from build123d import *

# Parameters (mm, degrees)
F0_R     = 4.7575
F0_R_2   = 1.5
F1_DEPTH = 3


with BuildPart() as f1:
    # F0 (on Front) → F1 (new body)
    with BuildSketch(Plane.XZ):
        with BuildLine():
            ThreePointArc((20.795049, 31.12199), (16.264046, 39.26488), (7.30225, 36.71089))
            ThreePointArc((7.30225, 36.71089), (4.659309, 40.877145), (0, 42.5))
            ThreePointArc((0, 42.5), (-4.659309, 40.877145), (-7.30225, 36.71089))
            ThreePointArc((-7.30225, 36.71089), (-16.264046, 39.26488), (-20.795049, 31.12199))
            ThreePointArc((-20.795049, 31.12199), (-25.609878, 32.199136), (-30.052038, 30.052038))
            ThreePointArc((-30.052038, 30.052038), (-32.199136, 25.609878), (-31.12199, 20.795049))
            ThreePointArc((-31.12199, 20.795049), (-39.26488, 16.264046), (-36.71089, 7.30225))
            ThreePointArc((-36.71089, 7.30225), (-40.877145, 4.659309), (-42.5, 0))
            ThreePointArc((-42.5, 0), (-40.877145, -4.659309), (-36.71089, -7.30225))
            ThreePointArc((-36.71089, -7.30225), (-39.26488, -16.264046), (-31.12199, -20.795049))
            ThreePointArc((-31.12199, -20.795049), (-32.199136, -25.609878), (-30.052038, -30.052038))
            ThreePointArc((-30.052038, -30.052038), (-25.609878, -32.199136), (-20.795049, -31.12199))
            ThreePointArc((-20.795049, -31.12199), (-16.264046, -39.26488), (-7.30225, -36.71089))
            ThreePointArc((-7.30225, -36.71089), (-4.659309, -40.877145), (0, -42.5))
            ThreePointArc((0, -42.5), (4.659309, -40.877145), (7.30225, -36.71089))
            ThreePointArc((7.30225, -36.71089), (16.264046, -39.26488), (20.795049, -31.12199))
            ThreePointArc((20.795049, -31.12199), (25.609878, -32.199136), (30.052038, -30.052038))
            ThreePointArc((30.052038, -30.052038), (32.199136, -25.609878), (31.12199, -20.795049))
            ThreePointArc((31.12199, -20.795049), (39.26488, -16.264046), (36.71089, -7.30225))
            ThreePointArc((36.71089, -7.30225), (40.877145, -4.659309), (42.5, 0))
            ThreePointArc((42.5, 0), (40.877145, 4.659309), (36.71089, 7.30225))
            ThreePointArc((36.71089, 7.30225), (39.26488, 16.264046), (31.12199, 20.795049))
            ThreePointArc((31.12199, 20.795049), (32.199136, 25.609878), (30.052038, 30.052038))
            ThreePointArc((30.052038, 30.052038), (25.609878, 32.199136), (20.795049, 31.12199))
        make_face()
        with BuildLine():
            ThreePointArc((-28.112798, -28.112798), (-28.112798, -21.384677), (-21.384677, -21.384677))
            ThreePointArc((-21.384677, -21.384677), (-20.35338, -22.928121), (-19.991237, -24.748737))
            ThreePointArc((-19.991237, -24.748737), (-22.928121, -29.144094), (-28.112798, -28.112798))
        make_face(mode=Mode.SUBTRACT)
        with Locations((-13.39392, -32.335784)):
            Circle(F0_R, mode=Mode.SUBTRACT)
        with Locations((-32.335784, -13.39392)):
            Circle(F0_R, mode=Mode.SUBTRACT)
        with BuildLine():
            ThreePointArc((0, -39.7575), (-4.7575, -35), (0, -30.2425))
            ThreePointArc((0, -30.2425), (3.364061, -31.635939), (4.7575, -35))
            ThreePointArc((4.7575, -35), (3.364061, -38.364061), (0, -39.7575))
        make_face(mode=Mode.SUBTRACT)
        with Locations((13.39392, -32.335784)):
            Circle(F0_R, mode=Mode.SUBTRACT)
        with Locations((0, -27)):
            Circle(F0_R_2, mode=Mode.SUBTRACT)
        with BuildLine():
            ThreePointArc((28.112798, -28.112798), (21.384677, -28.112798), (21.384677, -21.384677))
            ThreePointArc((21.384677, -21.384677), (26.569354, -20.35338), (29.506237, -24.748737))
            ThreePointArc((29.506237, -24.748737), (29.144094, -26.569354), (28.112798, -28.112798))
        make_face(mode=Mode.SUBTRACT)
        with Locations((32.335784, -13.39392)):
            Circle(F0_R, mode=Mode.SUBTRACT)
        with BuildLine():
            ThreePointArc((-39.7575, 0), (-35, 4.7575), (-30.2425, 0))
            ThreePointArc((-30.2425, 0), (-35, -4.7575), (-39.7575, 0))
        make_face(mode=Mode.SUBTRACT)
        with Locations((-27, 0)):
            Circle(F0_R_2, mode=Mode.SUBTRACT)
        with Locations((-32.335784, 13.39392)):
            Circle(F0_R, mode=Mode.SUBTRACT)
        with BuildLine():
            ThreePointArc((-19.991237, 24.748737), (-20.35338, 22.928121), (-21.384677, 21.384677))
            ThreePointArc((-21.384677, 21.384677), (-28.112798, 21.384677), (-28.112798, 28.112798))
            ThreePointArc((-28.112798, 28.112798), (-22.928121, 29.144094), (-19.991237, 24.748737))
        make_face(mode=Mode.SUBTRACT)
        with Locations((-13.39392, 32.335784)):
            Circle(F0_R, mode=Mode.SUBTRACT)
        with BuildLine():
            ThreePointArc((0, 11), (4.209518, 10.162675), (7.778175, 7.778175))
            ThreePointArc((7.778175, 7.778175), (10.162675, 4.209518), (11, 0))
            ThreePointArc((11, 0), (10.162675, -4.209518), (7.778175, -7.778175))
            ThreePointArc((7.778175, -7.778175), (4.209518, -10.162675), (0, -11))
            ThreePointArc((0, -11), (-4.209518, -10.162675), (-7.778175, -7.778175))
            ThreePointArc((-7.778175, -7.778175), (-10.162675, -4.209518), (-11, 0))
            ThreePointArc((-11, 0), (-10.162675, 4.209518), (-7.778175, 7.778175))
            ThreePointArc((-7.778175, 7.778175), (-4.209518, 10.162675), (0, 11))
        make_face(mode=Mode.SUBTRACT)
        with Locations((27, 0)):
            Circle(F0_R_2, mode=Mode.SUBTRACT)
        with BuildLine():
            ThreePointArc((39.7575, 0), (35, -4.7575), (30.2425, 0))
            ThreePointArc((30.2425, 0), (35, 4.7575), (39.7575, 0))
        make_face(mode=Mode.SUBTRACT)
        with Locations((32.335784, 13.39392)):
            Circle(F0_R, mode=Mode.SUBTRACT)
        with Locations((0, 27)):
            Circle(F0_R_2, mode=Mode.SUBTRACT)
        with BuildLine():
            ThreePointArc((0, 39.7575), (3.364061, 38.364061), (4.7575, 35))
            ThreePointArc((4.7575, 35), (3.364061, 31.635939), (0, 30.2425))
            ThreePointArc((0, 30.2425), (-4.7575, 35), (0, 39.7575))
        make_face(mode=Mode.SUBTRACT)
        with Locations((13.39392, 32.335784)):
            Circle(F0_R, mode=Mode.SUBTRACT)
        with BuildLine():
            ThreePointArc((21.384677, 21.384677), (21.384677, 28.112798), (28.112798, 28.112798))
            ThreePointArc((28.112798, 28.112798), (29.144094, 26.569354), (29.506237, 24.748737))
            ThreePointArc((29.506237, 24.748737), (26.569354, 20.35338), (21.384677, 21.384677))
        make_face(mode=Mode.SUBTRACT)
    extrude(amount=F1_DEPTH)


solid = f1.part
Verification items for the finished model (mm, model axes). Round coordinates to 2 decimals unless told otherwise and drop trailing zeros. Order: outer loops, then holes, each group sorted by start corner. A loop starts at its lowest first (then second) coordinate and runs counter-clockwise, first axis right, second up. Notation, with made-up numbers: (80, 7.25) -> (88, 7.25) arc R15 cw to (88, 32.25) -> close; hole circle Ø5 at (41, 60.5). An arc over 180 degrees is marked (long way). Put each result on its own line as item: value.
1) Section check A-A (x = 14). Record the cut outline in (y, z).
Final values:
outline: (-3, -39.81) -> (0, -39.81) -> (0, -37.05) -> (-3, -37.05) -> close; (-3, -27.62) -> (0, -27.62) -> (0, 27.62) -> (-3, 27.62) -> close; (-3, 37.05) -> (0, 37.05) -> (0, 39.81) -> (-3, 39.81) -> close
2) Section check B-B (x = -35). Record the cut outline in (y, z), then the cut area to 3 significant figures.
Final values:
outline: (-3, -20.4) -> (0, -20.4) -> (0, -17.34) -> (-3, -17.34) -> close; (-3, -9.45) -> (0, -9.45) -> (0, -4.76) -> (-3, -4.76) -> close; (-3, 4.76) -> (0, 4.76) -> (0, 9.45) -> (-3, 9.45) -> close; (-3, 17.34) -> (0, 17.34) -> (0, 20.4) -> (-3, 20.4) -> close
area: 46.6 mm^2
3) Depth check by flat-ended pin: pin 1 (1.5 mm diameter, centred on x = 16, y = -2, fed in from +Z). Enter the tip coordinate at first touch or a pass-through.
Final values:
pin 1: stops at z = 39.6
4) Section check D-D (z = 2.5). Record the cut outline in (x, y).
Final values:
outline: (-42.07, -3) -> (-39.05, -3) -> (-39.05, 0) -> (-42.07, 0) -> close; (-30.95, -3) -> (-10.71, -3) -> (-10.71, 0) -> (-30.95, 0) -> close; (10.71, -3) -> (30.95, -3) -> (30.95, 0) -> (10.71, 0) -> close; (39.05, -3) -> (42.07, -3) -> (42.07, 0) -> (39.05, 0) -> close
5) Mould release check, pull along Z, two halves, no side actions. Record for faces 1 (the flat face through (9, -3, -9)), 2 (the cylindrical face through (-28.5, -1.48, 0.07)): +Z half, -Z half, draft (parallel to the pull), parting line (faces both ways), or undercut.
Final values:
face 1: draft
face 2: undercut
6) Material ranges on line 1 (X direction, y = -2, z = 1); line 2 (Z direction, x = 27, y = -1.85); line 3 (Z direction, x = -4, y = -0.3), recorded low to high.
Final values:
line 1: x = -42.43 to -39.65, -30.35 to -28.12, -25.88 to -10.95, 10.95 to 25.88, 28.12 to 30.35, 39.65 to 42.43
line 2: z = -31.9 to -28.94, -20.56 to -1.5, 1.5 to 20.56, 28.94 to 31.9
line 3: z = -41.34 to -37.58, -32.42 to -10.25, 10.25 to 32.42, 37.58 to 41.34
7) Section check C-C (z = 23). Record the cut outline in (x, y), then the cut area to 3 significant figures.
Final values:
outline: (-32.04, -3) -> (-29.17, -3) -> (-29.17, 0) -> (-32.04, 0) -> close; (-20.32, -3) -> (20.32, -3) -> (20.32, 0) -> (-20.32, 0) -> close; (29.17, -3) -> (32.04, -3) -> (32.04, 0) -> (29.17, 0) -> close
area: 139 mm^2
